Build history of the part. All positions in model axes, mm. Face numbers are marked on the shaded views. A direction names the side the tool comes from. Round coordinates to 2 decimals unless told otherwise and drop trailing zeros. Write each loop counter-clockwise with the first axis right and the second up, starting at its lowest first coordinate (ties: lowest second). Pieces come first, ordered by that corner, then holes. Notation, with made-up numbers: M 18.5,27.5 L 29.5,27.5 A30 ccw 29.5,66.5 Z; hole C 43.5,-35 d7. An arc over 180 degrees is marked long. Use a Markdown table: item, result.
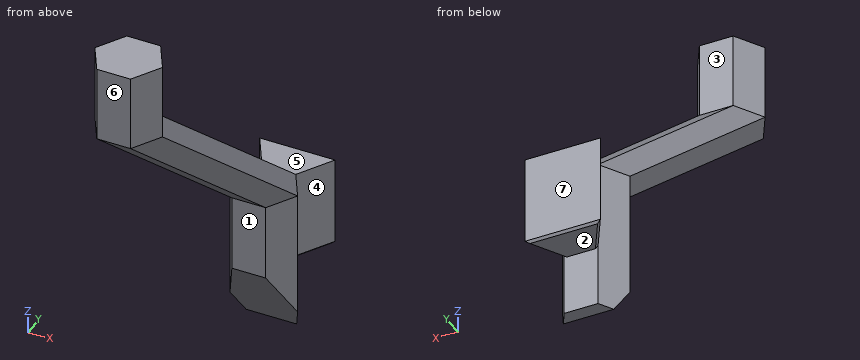
from build123d import *

# Parameters (mm, degrees)
BOSS_EXTRUDE1_DEPTH = 25.4
BOSS_EXTRUDE2_DEPTH = 12.7
BOSS_EXTRUDE3_DEPTH = 25.4
CHAMFER1_SIZE       = 7.46
CHAMFER1_SIZE2      = 12.54
CUT_EXTRUDE1_DEPTH  = 10.16
CHAMFER7_SIZE       = 0.381


with BuildPart() as part:
    # Sketch1 → Boss-Extrude1 (new body)
    with BuildSketch(Plane.XY):
        Polygon((5.715, 0), (2.8575, 4.949335183), (-2.8575, 4.949335183), (-5.715, 0), (-2.8575, -4.949335183), (2.8575, -4.949335183), align=None)
    extrude(amount=BOSS_EXTRUDE1_DEPTH)



with BuildPart() as body_2:
    # Sketch2 → Boss-Extrude2 (new body)
    with BuildSketch(Plane.XY.offset(63.5)):
        Polygon((-2.8575, -49.399335183), (2.8575, -49.399335183), (5.715, -44.45), (2.8575, -39.500664817), (-2.8575, -39.500664817), (-5.715, -44.45), align=None)
    extrude(amount=BOSS_EXTRUDE2_DEPTH)


with BuildPart() as part_1:
    add(part.part)

    add(body_2.part)  # loft1 joins it to this body
    # loft from a face of the part (loft1)
    loft([part_1.faces().sort_by_distance((0, 0, 25.4))[0], part_1.faces().sort_by_distance((0, -44.45, 63.5))[0]])

    # Sketch4 → Boss-Extrude3 (add)
    with BuildSketch(Plane(origin=(0, 0, 0), x_dir=(-1, 0, 0), z_dir=(0, 0, -1))):
        Polygon((2.8575, 4.949335183), (6.377027241, 11.045335183), (-6.377027241, 11.045335183), (-2.8575, 4.949335183), align=None)
    extrude(amount=-BOSS_EXTRUDE3_DEPTH)

    # Chamfer1
    chamfer1_edges = [part_1.edges().sort_by_distance(p)[0] for p in [
        (0, -4.949335183, 0),
    ]]
    chamfer1_side = [part_1.faces().sort_by_distance(p)[0] for p in [
        (0, 3.343943544, 0),
    ]]
    chamfer(chamfer1_edges, length=CHAMFER1_SIZE, length2=CHAMFER1_SIZE2, reference=chamfer1_side[0])

    # Sketch8 → Cut-Extrude1 (cut)
    with BuildSketch(Plane(origin=(0, 0, 0), x_dir=(-1, 0, 0), z_dir=(0, 0, -1))):
        Polygon((-6.377027241, 11.045335183), (6.377027241, 11.045335183), (2.8575, 4.949335183), (-2.8575, 4.949335183), align=None)
    extrude(amount=-CUT_EXTRUDE1_DEPTH, mode=Mode.SUBTRACT)

    # Chamfer7
    chamfer7_edges = [part_1.edges().sort_by_distance(p)[0] for p in [
        (4.61726362, 7.997335183, 10.16),
        (0, 11.045335183, 10.16),
        (-4.61726362, 7.997335183, 10.16),
    ]]
    chamfer(chamfer7_edges, length=CHAMFER7_SIZE)


solid = part_1.part
Q1. Cut at A-A on x = 0.25. Give the cut face in (y, z), and give its area (3 significant figures).
Response values:
| item | result |
|---|---|
| outline | M -49.4,63.5 L -4.95,25.4 L -4.95,12.54 L 2.51,0 L 4.95,0 L 4.95,10.16 L 10.66,10.16 L 11.05,10.54 L 11.05,25.4 L 4.95,25.4 L -39.5,63.5 L -39.5,76.2 L -49.4,76.2 Z |
| area | 800 mm2 |
Q2. Which spindle directions (+Z, -Z, +X, -X, +Y, -Y) get a long thin tool onto all of the face, cutting with end or side? Do the marked faces 1, 2 and 3. Say none if no direction does.
Response values:
| item | result |
|---|---|
| face 1 | -Z, +X, -X, -Y |
| face 2 | -Z, +X, -X, +Y |
| face 3 | +Z, +X, -X, +Y |
Q3. Drop flat-ended pins along their axis: P1, Ø3, axis at x = -0.5, z = 67.5, coming from the +Y side; P2, Ø1, axis at x = -2.5, z = 30.5, coming from the -Y side; P3, Ø4.5, axis at x = -1, z = 17.5, coming from the -Y side; P4, Ø6, axis at x = 1.5, z = 27, coming from the +Y side. Give the stop position or say it passes through.
Response values:
| item | result |
|---|---|
| P1 | stops at y = -39.5 |
| P2 | stops at y = -11.48 |
| P3 | stops at y = -4.95 |
| P4 | stops at y = 11.05 |
Q4. Cut at C-C on z = 9. Give the cut face in (x, y) (1 decimal), and give its area (3 significant figures).
Response values:
| item | result |
|---|---|
| outline | M -5.7,0 L -4.1,-2.8 L 4.1,-2.8 L 5.7,0 L 2.9,4.9 L -2.9,4.9 Z |
| area | 70.3 mm2 |
Q5. Cut at B-B on z = 24. Give the cut face in (x, y) (1 decimal), and give its area (3 significant figures).
Response values:
| item | result |
|---|---|
| outline | M -6.4,11 L -2.9,4.9 L -5.7,0 L -2.9,-4.9 L 2.9,-4.9 L 5.7,0 L 2.9,4.9 L 6.4,11 Z |
| area | 141 mm2 |
Q6. Two-plate mould, pull along Y, no slides. Class the marked faces 4, 5, 6 and 7: +Y half, -Y half, draft (parallel to the pull), parting line (faces both ways), or undercut.
Response values:
| item | result |
|---|---|
| face 4 | undercut |
| face 5 | draft |
| face 6 | -Y half |
| face 7 | +Y half |
Q7. Drill centre lines: L1, parallel to Y at x = 1.5, z = 19.5; L2, parallel to Z at x = -0.75, y = -8; L3, parallel to Z at x = 2.5, y = -34. Where is each one in solid material? Low to high.
Response values:
| item | result |
|---|---|
| L1 | y = -4.95 to 11.05 |
| L2 | z = 28.01 to 36.5 |
| L3 | z = 50.3 to 58.79 |
